from build123d import *

# Parameters (mm, degrees)
SKETCH1_W           = 25
SKETCH1_H           = 112.5
SKETCH1_H_2         = 25
SKETCH1_W_2         = 112.5
BOSS_EXTRUDE1_DEPTH = 10
SKETCH2_R           = 50.8
BOSS_EXTRUDE2_DEPTH = 15


with BuildPart() as part:
    # Sketch1 → Boss-Extrude1 (new body)
    with BuildSketch(Plane(origin=(0, 0, 0), x_dir=(1, 0, 0), z_dir=(0, 1, 0))):
        with Locations((0, 68.75)):
            Rectangle(SKETCH1_W, SKETCH1_H)
        Rectangle(SKETCH1_W, SKETCH1_H_2)
        with Locations((0, -68.75)):
            Rectangle(SKETCH1_W, SKETCH1_H)
        with Locations((68.75, 0)):
            Rectangle(SKETCH1_W_2, SKETCH1_H_2)
        with Locations((-68.75, 0)):
            Rectangle(SKETCH1_W_2, SKETCH1_H_2)
    extrude(amount=BOSS_EXTRUDE1_DEPTH)

    # Sketch2 → Boss-Extrude2 (add)
    with BuildSketch(Plane(origin=(0, 10, 0), x_dir=(1, 0, 0), z_dir=(0, 1, 0))):
        with Locations(Location((0, 125, 0), (0, 0, 255.755338046))):
            Circle(SKETCH2_R)
        with Locations(Location((125, 0, 0), (0, 0, 165.755338046))):
            Circle(SKETCH2_R)
        with Locations(Location((0, -125, 0), (0, 0, 75.755338046))):
            Circle(SKETCH2_R)
        with Locations(Location((-125, 0, 0), (0, 0, 14.244661954))):
            Circle(SKETCH2_R)
    extrude(amount=BOSS_EXTRUDE2_DEPTH)


solid = part.part
Design review of the part built by this model. Coordinates are the model's own, in mm. A direction names the side the tool comes from. Coordinates: 2 decimals unless noted, no trailing zeros. Loops run counter-clockwise (first coordinate to the right, second up) from the corner with the lowest first, then second, coordinate; pieces in that order, holes last. Notation, with made-up numbers: (74, 54.5) -> (93, 54.5) arc R28 ccw to (93, 89.5) -> close; hole circle Ø8 at (55.5, -35). An arc over 180 degrees is marked (long way). Use a Markdown table: item, result. Add a question column.
Item 1: Machinability: for faces 1 (the flat face through (-12.5, 5, 68)), 2 (the flat face through (0, 5, 125)), 3 (the flat face through (0, 5, -125)), 4 (the flat face through (-12.5, 5, -70)), which of the approach directions +Z, -Z, +X, -X, +Y, -Y give a long, thin tool a straight path to every point of the face, cutting with its end or side? Answer none if there is none.
Item 2: We need section A-A, the plane z = -39. Write out the cut boundary in (x, y), and give its area (3 significant figures).
Item 3: We need section C-C, the plane y = 4.5. Write out the cut boundary in (x, z), and give its area (3 significant figures).
Item 4: Wall thickness on L1, parallel to Z at x = 44, y = 5; L2, parallel to X at y = 11, z = 128; L3, parallel to Z at x = -14, y = 21.25: over which ranges is each line inside the solid? List them lowest first. Write a range as from..to.
Item 5: The part is to be moulded in two halves that separate along X. For faces 5 (the cylindrical face through (-81.79, 17.4, -26.71)), 6 (the flat face through (12.5, 5, 70)), 7 (the flat face through (68, 5, -12.5)), say which applies: +X half, -X half, draft (parallel to the pull), parting line (faces both ways), or undercut.
Item 6: We need section D-D, the plane x = 44. Write out the cut boundary in (y, z).
Item 7: Clearance check with flat-ended pins moving along their axes: P1, Ø3, axis at x = -75.5, y = 5, coming from the +Z side; P2, Ø12, axis at x = 130.5, y = 17, coming from the +Z side; P3, Ø12, axis at x = -83, y = 17.5, coming from the +Z side. State where each tip first meets the part, or that it passes through.
Item 8: We need section B-B, the plane x = 0. Write out the cut boundary in (y, z).
Numbers:
| question | item | result |
|---|---|---|
| 1 | face 1 | +Z, -X, -Y |
| 1 | face 2 | +Z, +X, -X, -Y |
| 1 | face 3 | -Z, +X, -X, -Y |
| 1 | face 4 | -Z, -X, -Y |
| 2 | outline | (-157.55, 10) -> (-92.45, 10) -> (-92.45, 25) -> (-157.55, 25) -> close; (-12.5, 0) -> (12.5, 0) -> (12.5, 10) -> (-12.5, 10) -> close; (92.45, 10) -> (157.55, 10) -> (157.55, 25) -> (92.45, 25) -> close |
| 2 | area | 2,200 mm^2 |
| 3 | outline | (-125, -12.5) -> (-12.5, -12.5) -> (-12.5, -125) -> (12.5, -125) -> (12.5, -12.5) -> (125, -12.5) -> (125, 12.5) -> (12.5, 12.5) -> (12.5, 125) -> (-12.5, 125) -> (-12.5, 12.5) -> (-125, 12.5) -> close |
| 3 | area | 11,900 mm^2 |
| 4 | L1 | z = -12.5..12.5 |
| 4 | L2 | x = -50.71..50.71 |
| 4 | L3 | z = -173.83..-76.17, 76.17..173.83 |
| 5 | face 5 | undercut |
| 5 | face 6 | +X half |
| 5 | face 7 | draft |
| 6 | outline | (0, -12.5) -> (10, -12.5) -> (10, 12.5) -> (0, 12.5) -> close; (10, -150.39) -> (25, -150.39) -> (25, -99.61) -> (10, -99.61) -> close; (10, 99.61) -> (25, 99.61) -> (25, 150.39) -> (10, 150.39) -> close |
| 7 | P1 | stops at z = 12.5 |
| 7 | P2 | stops at z = 50.8 |
| 7 | P3 | stops at z = 35.84 |
| 8 | outline | (0, -125) -> (10, -125) -> (10, -175.8) -> (25, -175.8) -> (25, -74.2) -> (10, -74.2) -> (10, 74.2) -> (25, 74.2) -> (25, 175.8) -> (10, 175.8) -> (10, 125) -> (0, 125) -> close |
